Study the drawing (mm; zero at the part's minimum x, y, z) and answer. Coordinates: 2 decimals unless noted, no trailing zeros. Order: outer loops, then holes, each group sorted by start corner. A loop starts at its lowest first (then second) coordinate and runs counter-clockwise, first axis right, second up. Notation, with made-up numbers: (6, 50.5) -> (26, 50.5) arc R33 ccw to (26, 79.5) -> close; hole circle Ø1 at (15.5, 78). An arc over 180 degrees is marked (long way). Answer in a Markdown table with one row per item. Add a question column.
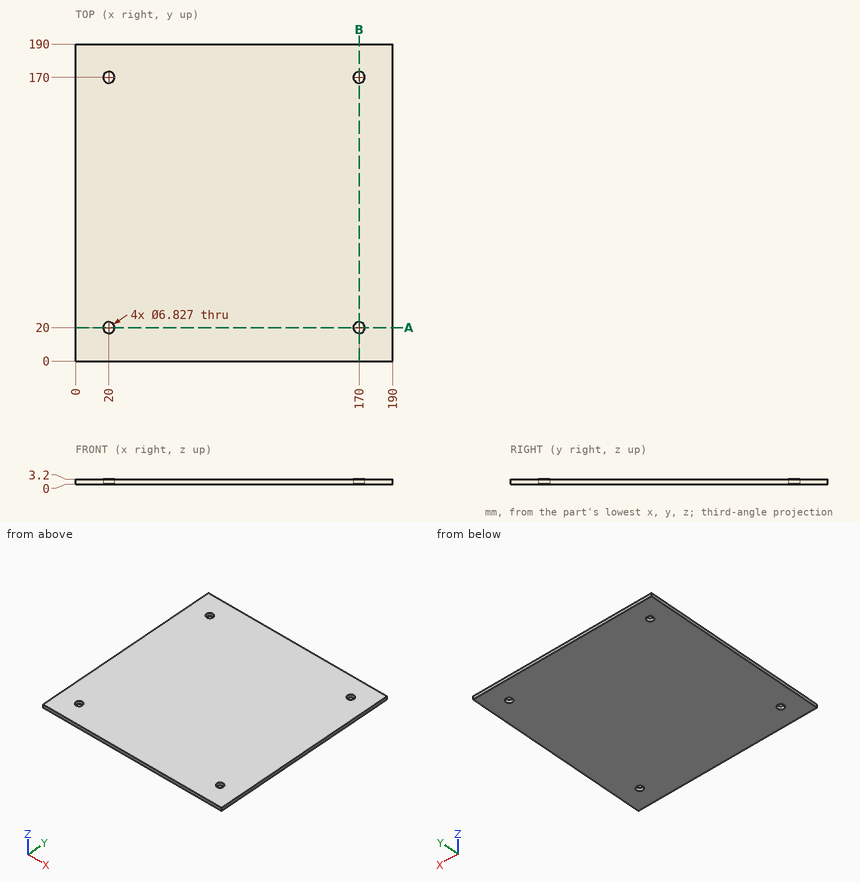
Q1. A cutting plane is placed at A-A (y = 20). Determine the outline of the cut face in (x, z).
Q2. Given pin 1 (9 mm diameter, centred on x = 20, y = 170, fed in from +Z), flat-ended and moving along its own axis, determine where the tip first touches the part or whether it passes through.
Q3. Straight lines are drawn through the part: line 1 (Y direction, x = 170, z = 1.35); line 2 (X direction, y = 167.5, z = 0.45) (1 decimal). For each, find the intervals that lie inside material, in ascending order.
Returned:
| question | item | result |
|---|---|---|
| 1 | outline | (0, 0) -> (16.59, 0) -> (16.59, 3.2) -> (0, 3.2) -> close; (23.41, 0) -> (166.59, 0) -> (166.59, 3.2) -> (23.41, 3.2) -> close; (173.41, 0) -> (190, 0) -> (190, 3.2) -> (173.41, 3.2) -> close |
| 2 | pin 1 | stops at z = 3.2 |
| 3 | line 1 | y = 0 to 16.59, 23.41 to 166.59, 173.41 to 190 |
| 3 | line 2 | x = 0 to 17.7, 22.3 to 167.7, 172.3 to 190 |
